Source: CAD feature listing. Evaluate the final solid. Frame: model axes, mm. Face numbers are marked on the shaded views. Round coordinates to 2 decimals unless told otherwise and drop trailing zeros. Loops run counter-clockwise (first coordinate to the right, second up) from the corner with the lowest first, then second, coordinate; pieces in that order, holes last. Notation, with made-up numbers: (-31.75, -8.5) -> (16.25, -8.5) arc R26 cw to (16.25, 7.5) -> close; hole circle Ø9 at (-13.75, -5). An arc over 180 degrees is marked (long way). Return JSON: item names as keys, results as strings. Group by question number.
```python
from build123d import *

# Parameters (mm, degrees)
SZKIC1_W                    = 32.48
SZKIC1_H                    = 5.8
DODANIE_WYCI_GNI_CIE1_DEPTH = 3.4
SZKIC2_W                    = 0.64
SZKIC2_H                    = 0.64
WYTNIJ_WYCI_GNI_CIE1_DEPTH  = 3.4
SZKIC3_W                    = 32.48
SZKIC3_H                    = 5.8
SZKIC3_W_2                  = 30.48
SZKIC3_H_2                  = 3.8
DODANIE_WYCI_GNI_CIE2_DEPTH = 8.1
SZKIC4_W                    = 1
SZKIC4_H                    = 1
WYTNIJ_WYCI_GNI_CIE2_DEPTH  = 3.4
ZAOKR_GLENIE1_R             = 1


with BuildPart() as part:
    # Szkic1 → Dodanie-wyciągnięcie1 (new body)
    with BuildSketch(Plane(origin=(0, 0, 0), x_dir=(1, 0, 0), z_dir=(0, 1, 0))):
        with Locations((-4.592060125, -1.597771029)):
            Rectangle(SZKIC1_W, SZKIC1_H)
    extrude(amount=DODANIE_WYCI_GNI_CIE1_DEPTH)

    # Szkic2 → Wytnij-wyciągnięcie1 (cut)
    with BuildSketch(Plane(origin=(0, 3.4, 0), x_dir=(1, 0, 0), z_dir=(0, 1, 0))):
        with Locations((-18.562060125, -1.597771029)):
            Rectangle(SZKIC2_W, SZKIC2_H)
        with Locations((-16.022060125, -1.597771029)):
            Rectangle(SZKIC2_W, SZKIC2_H)
        with Locations((-13.482060125, -1.597771029)):
            Rectangle(SZKIC2_W, SZKIC2_H)
        with Locations((-10.942060125, -1.597771029)):
            Rectangle(SZKIC2_W, SZKIC2_H)
        with Locations((-8.402060125, -1.597771029)):
            Rectangle(SZKIC2_W, SZKIC2_H)
        with Locations((-5.862060125, -1.597771029)):
            Rectangle(SZKIC2_W, SZKIC2_H)
        with Locations((-3.322060125, -1.597771029)):
            Rectangle(SZKIC2_W, SZKIC2_H)
        with Locations((-0.782060125, -1.597771029)):
            Rectangle(SZKIC2_W, SZKIC2_H)
        with Locations((1.757939875, -1.597771029)):
            Rectangle(SZKIC2_W, SZKIC2_H)
        with Locations((4.297939875, -1.597771029)):
            Rectangle(SZKIC2_W, SZKIC2_H)
        with Locations((6.837939875, -1.597771029)):
            Rectangle(SZKIC2_W, SZKIC2_H)
        with Locations((9.377939875, -1.597771029)):
            Rectangle(SZKIC2_W, SZKIC2_H)
    extrude(amount=-WYTNIJ_WYCI_GNI_CIE1_DEPTH, mode=Mode.SUBTRACT)

    # Szkic3 → Dodanie-wyciągnięcie2 (add)
    with BuildSketch(Plane(origin=(0, 3.4, 0), x_dir=(1, 0, 0), z_dir=(0, 1, 0))):
        with Locations((-4.592060125, -1.597771029)):
            Rectangle(SZKIC3_W, SZKIC3_H)
        with Locations((-4.592060125, -1.597771029)):
            Rectangle(SZKIC3_W_2, SZKIC3_H_2, mode=Mode.SUBTRACT)
    extrude(amount=DODANIE_WYCI_GNI_CIE2_DEPTH)

    # Szkic4 → Wytnij-wyciągnięcie2 (cut)
    with BuildSketch(Plane(origin=(0, 11.5, 0), x_dir=(1, 0, 0), z_dir=(0, 1, 0))):
        with Locations((-20.332060125, -2.997771029)):
            Rectangle(SZKIC4_W, SZKIC4_H)
        with Locations((-19.332060125, -3.997771029)):
            Rectangle(SZKIC4_W, SZKIC4_H)
        with Locations((-20.332060125, -0.197771029)):
            Rectangle(SZKIC4_W, SZKIC4_H)
        with Locations((-19.332060125, 0.802228971)):
            Rectangle(SZKIC4_W, SZKIC4_H)
        with Locations((10.147939875, 0.802228971)):
            Rectangle(SZKIC4_W, SZKIC4_H)
        with Locations((11.147939875, -0.197771029)):
            Rectangle(SZKIC4_W, SZKIC4_H)
        with Locations((11.147939875, -2.997771029)):
            Rectangle(SZKIC4_W, SZKIC4_H)
        with Locations((10.147939875, -3.997771029)):
            Rectangle(SZKIC4_W, SZKIC4_H)
    extrude(amount=-WYTNIJ_WYCI_GNI_CIE2_DEPTH, mode=Mode.SUBTRACT)

    # Zaokrąglenie1
    zaokr_glenie1_edges = [part.edges().sort_by_distance(p)[0] for p in [
        (11.147939875, 8.1, 2.497771029),
        (11.147939875, 8.1, 0.697771029),
        (9.647939875, 8.1, -0.802228971),
        (9.647939875, 8.1, 3.997771029),
        (-18.832060125, 8.1, -0.802228971),
        (-20.332060125, 8.1, 0.697771029),
        (-20.332060125, 8.1, 2.497771029),
        (-18.832060125, 8.1, 3.997771029),
    ]]
    fillet(zaokr_glenie1_edges, radius=ZAOKR_GLENIE1_R - 0.0001)  # a hair under: the kernel refuses the full size


solid = part.part
```
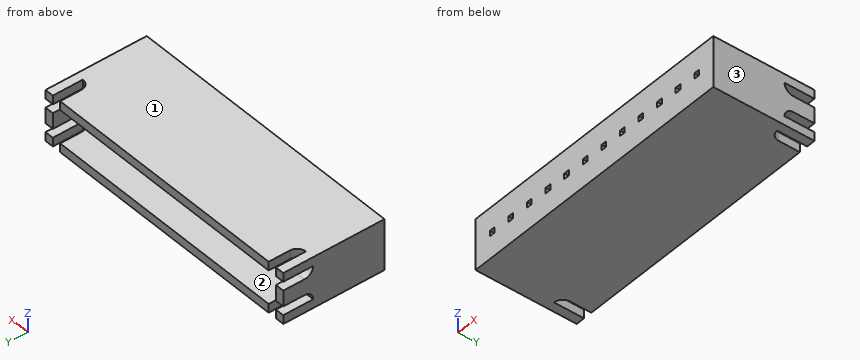
(1) Pin query (flat end, axial travel): pin 1 (1.5 mm diameter, centred on x = -6.5, z = 2.5, fed in from +Y). Return the tip coordinate at first contact, or that it passes through.
(2) Mould query, pull axis Z, two halves, no side actions, for the marked faces 1, 2 and 3. Classes: released by +Z, released by -Z, zero draft, split by the parting line, or undercut.
(3) Cut plane B-B (x = 7.5). Return loops of the section in (y, z).
(4) Ray query, line 1 (Z direction, x = -1, y = 1.5); line 2 (X direction, y = 6.5, z = 3.15); line 3 (Z direction, x = -18, y = 4). Return the intervals inside material, ascending.
(5) Cut plane D-D (z = 2.85). Return loops of the section in (x, y).
(6) Cut plane C-C (y = 8.75). Count the separate pieces of the cut face and the enclosed holes in it, and give its area (3 significant figures).
(7) Cut plane A-A (y = 4.75). Return loops of the section in (x, z), and give its area (3 significant figures).
Answers follow:
{
 "1": {"pin 1": "y = 3.4"},
 "2": {"face 1": "released by +Z", "face 2": "undercut", "face 3": "zero draft"},
 "3": {"outline": "(0, -1.3) -> (11.5, -1.3) -> (11.5, -0.3) -> (3.4, -0.3) -> (3.4, 3.5) -> (11.5, 3.5) -> (11.5, 4.5) -> (0, 4.5) -> close"},
 "4": {"line 1": "-1.3 to 1.28, 1.92 to 4.5", "line 2": "-20.83 to -19.83, 10.65 to 11.65", "line 3": "-1.3 to -0.3, 3.5 to 4.5"},
 "5": {"outline": "(-20.83, 0) -> (11.65, 0) -> (11.65, 8.34) -> (10.65, 8.34) -> (10.65, 3.4) -> (-19.83, 3.4) -> (-19.83, 8.34) -> (-20.83, 8.34) -> close"},
 "6": {"separate pieces": "8", "enclosed holes": "0", "area": "65.1 mm^2"},
 "7": {"outline": "(-20.83, -1.3) -> (11.65, -1.3) -> (11.65, 4.5) -> (-20.83, 4.5) -> close; hole (-19.83, -0.3) -> (10.65, -0.3) -> (10.65, 3.5) -> (-19.83, 3.5) -> close", "area": "72.6 mm^2"}
}
